Could you check a few things on this drawing? It's one solid part, dimensions in mm from its lowest x, y, z. A direction names the side the tool comes from. Give positions to 0.01 mm unless a question says otherwise; leave off trailing zeros. Loops run counter-clockwise (first coordinate to the right, second up) from the corner with the lowest first, then second, coordinate; pieces in that order, holes last.
Q1. I'm going to push flat-ended pins straight in: P1, Ø11, axis at x = 9, y = 50.5, coming from the +Z side; P2, Ø6, axis at x = 7, y = 15.5, coming from the +Z side; P3, Ø6, axis at x = 10, y = 49.75, coming from the +Z side; P4, Ø4.5, axis at x = 10, y = 8.5, coming from the -Z side. Where does each tip first touch, or does it pass through?
Q2. For the marked faces 1, 2 and 3, which set-ups out of +Z, -Z, +X, -X, +Y, -Y let a thin tool reach every point of the face, with its end or its side?
Q3. Suppose I cut it at A-A (z = 6.75). List the corners of the cut face in (x, y) for me.
Q4. I need wall thicknesses on probe 1 along Y at (x, z) = (10, 1.85); probe 2 along Y at (x, z) = (10, 2.7); probe 3 along Z at (x, y) = (14.75, 54). Which ranges of each line are inside material? Lowest first, please.
Q5. Thinking about a two-plate mould opening in Y: for the marked faces 4, 5 and 6, which applies, pulls with the +Y half, pulls with the -Y half, needs draft (parallel to the pull), parting line crosses it, or undercut?
Q6. Suppose I cut it at C-C (x = 8.25). Count the separate pieces of the cut face and the enclosed holes in it.
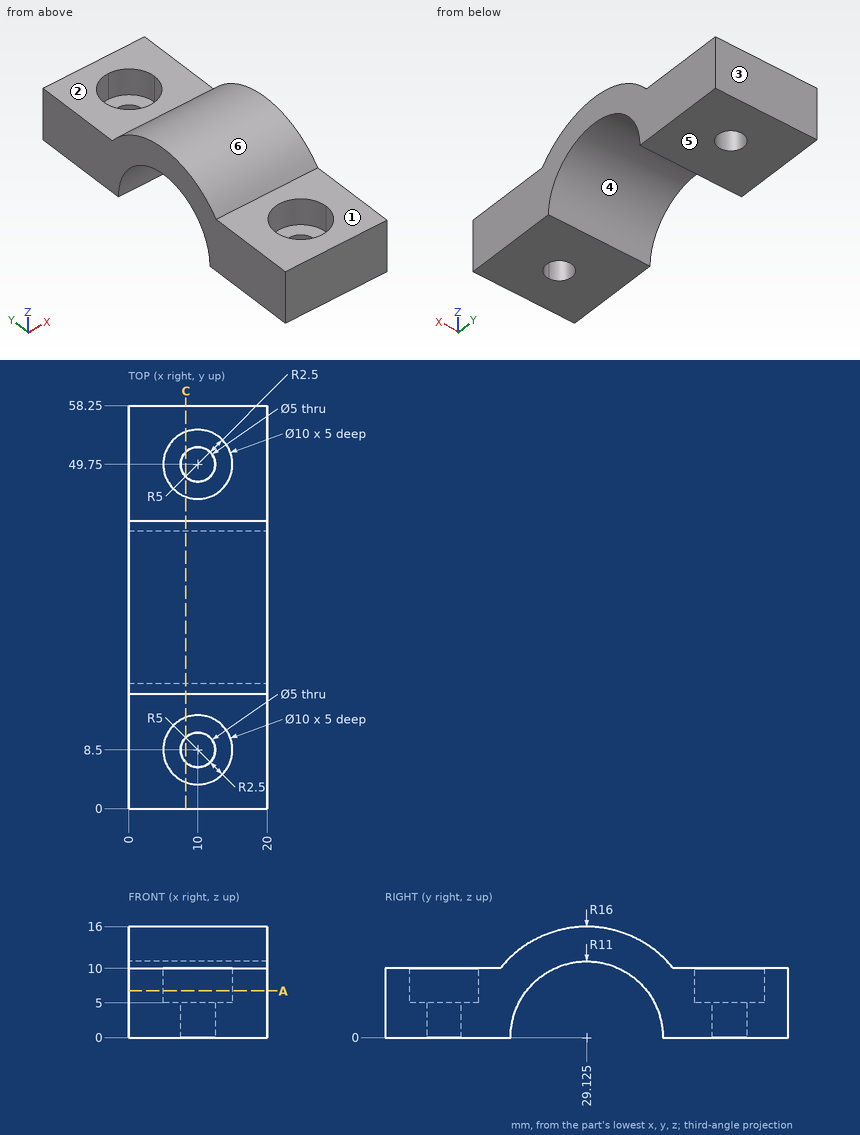
Solutions:
1. P1: stops at z = 10
1. P2: stops at z = 11.96
1. P3: stops at z = 5
1. P4: passes through
2. face 1: +Z, +X, -X, -Y
2. face 2: +Z, +X, -X, +Y
2. face 3: +Z, -Z, +X, -X, +Y
3. outline: (0, 0) - (20, 0) - (20, 20.44) - (0, 20.44) - close; (0, 37.81) - (20, 37.81) - (20, 58.25) - (0, 58.25) - close; hole circle Ø10 at (10, 8.5); hole circle Ø10 at (10, 49.75)
4. probe 1: y = 0 to 6, 11 to 18.28, 39.97 to 47.25, 52.25 to 58.25
4. probe 2: y = 0 to 6, 11 to 18.46, 39.79 to 47.25, 52.25 to 58.25
4. probe 3: z = 0 to 10
5. face 4: undercut
5. face 5: needs draft
5. face 6: parting line crosses it
6. separate pieces: 3
6. enclosed holes: 0
